Work out the finished part from the listing and answer in its coordinate system (mm). A direction names the side the tool comes from. Give positions to 0.01 mm unless a question says otherwise; leave off trailing zeros. Write each loop counter-clockwise with the first axis right and the second up, starting at its lowest first coordinate (ties: lowest second). Pieces come first, ordered by that corner, then holes.
1) Find section A-A (y = -11). Determine the outline of the cut face in (x, z).
2) Find section B-B (x = -92). Determine the outline of the cut face in (y, z), plus the area to 3 significant figures.
3) Straight lines are drawn through the part: probe 1 along Y at (x, z) = (-18, -18); probe 2 along X at (y, z) = (-7, -22); probe 3 along X at (y, z) = (-15.5, -32). For each, find the intervals that lie inside material, in ascending order.
4) Given pin 1 Ø12 at (x, y) = (-22, -35) entering from -Z; pin 2 Ø6 at (x, z) = (-67.5, -25.5) entering from -Y; pin 3 Ø7.5 at (y, z) = (-14, -30.5) entering from +X; pin 4 Ø10.5 at (x, z) = (-27.72, -17.76) entering from +Y, each flat-ended and moving along its own axis, determine where each tip first touches the part or whether it passes through.
5) A tool of negligible diameter and unlimited length cuts with its end or side. For faces 4 (the face through (-107, -46, -29)), 5 (the face through (-60, -3, -22)), 6 (the face through (-47, 0, -28)), from which of +Z, -Z, +X, -X, +Y, -Y can it reach the whole face along a straight path? Write none if from no direction.
6) Determine the mould class of faces 1 (the face through (-70.77, -1.48, -29.35)), 2 (the face through (-15.8, -17.5, -21.7)), 3 (the face through (-104.204, -24, -29)) for opening direction Z: pulls with the +Z half, pulls with the -Z half, needs draft (parallel to the pull), parting line crosses it, or undercut.
Autodesk Inventor part; units mm, degrees
ref_plane "YZ Plane" through (0, 0, 0) normal (1, 0, 0) x (0, 1, 0)
ref_plane "XZ Plane" through (0, 0, 0) normal (0, 1, 0) x (-1, 0, 0)
ref_plane "XY Plane" through (0, 0, 0) normal (0, 0, 1) x (1, 0, 0)
sketch "Sketch1" plane through (0, 0, 0) normal (0, 1, 0) x (-1, 0, 0)
  circle A0 centre (92.6541, -28.2127) radius 6.05
  circle A1 centre (65.1803, -27.0368) radius 6.05
  circle A2 centre (45.4573, -23.7633) radius 6.05
  circle A3 centre (92.6541, -28.2127) radius 7.55
  circle A4 centre (65.1803, -27.0368) radius 7.55
  circle A5 centre (45.4573, -23.7633) radius 7.55
  circle A6 centre (92.6541, -28.2127) radius 4
  circle A7 centre (45.4573, -23.7633) radius 4
  line L0 (92.6541, -28.2127) -> (100.2041, -28.2127)
  line L1 (70.678, -35.6025) -> (39.5208, -30.4313)
  line L2 (60.2143, -34.3811) -> (122.676, -37.0546)
  line L3 (51.451, -33.7618) -> (1.5927, -16.8916)
  line L4 (51.8932, -17.9704) -> (4.2209, -1.8399)
  circle A8 centre (27.7249, -17.7633) radius 4
  circle A9 centre (27.7249, -17.7633) radius 6.05
  circle A10 centre (27.7249, -17.7633) radius 7.55
  line L5 (27.7249, -17.7633) -> (20.1749, -17.7633)
  line L6 (20.1749, -17.7633) -> (16.1749, -17.7633)
  line L7 (16.1749, -17.7633) -> (10.1749, -17.7633)
  line L8 (10.1749, -17.7633) -> (10.1749, -19.7955)
  line L9 (10.1749, -19.7955) -> (10.1749, -3.8545)
  line L10 (13.1749, -17.7633) -> (13.1749, -20.8106)
  line L11 (13.1749, -20.8106) -> (13.1749, -4.8696)
  line L12 (13.1749, -20.8106) -> (13.1749, -16.8106)
  line L13 (13.1749, -4.8696) -> (13.1749, -8.8696)
  circle A11 centre (13.1749, -16.8106) radius 1
  circle A12 centre (13.1749, -8.8696) radius 1
  line L14 (16.1749, -17.7633) -> (16.1749, -21.8257)
  line L15 (16.1749, -17.7633) -> (16.1749, -5.8847)
  line L16 (114.6217, -21.596) -> (60.8612, -19.295)
  line L17 (100.2041, -28.2127) -> (104.2041, -28.2127)
  line L18 (104.2041, -28.2127) -> (110.2041, -28.2127)
  line L19 (107.2041, -28.2127) -> (107.2041, -21.2785)
  line L20 (107.2041, -28.2127) -> (107.2041, -36.3923)
  line L21 (107.2041, -36.3923) -> (107.2041, -28.3923)
  line L22 (107.2041, -21.2785) -> (107.2041, -25.2785)
  circle A13 centre (107.2041, -32.3923) radius 1
  circle A14 centre (107.2041, -25.2785) radius 1
  line L23 (110.2041, -28.2127) -> (110.2041, -36.5208)
  line L24 (104.2041, -28.2127) -> (104.2041, -36.2639)
  line L25 (104.2041, -28.2127) -> (104.2041, -21.1501)
  line L26 (110.2041, -28.2127) -> (110.2041, -21.4069)
  line L27 (75.2254, -21.0507) -> (39.3363, -15.0941)
  line L28 (65.1803, -27.0368) -> (45.4573, -27.0368)
  line L29 (55.3188, -33.0533) -> (55.3188, -17.7467)
  circle A15 centre (55.3188, -25.4) radius 1
  circle A16 centre (55.3188, -25.4) radius 2.55
  circle A17 centre (65.1803, -27.0368) radius 4
  point P0 (43.6173, -31.1112)
  point P1 (64.3979, -34.5602)
  point P2 (65.9627, -19.5133)
  point P3 (66.4165, -19.5886)
  point P4 (65.5031, -19.4937)
  point P5 (47.2973, -16.4154)
  point P6 (47.8772, -16.6116)
  point P7 (46.6935, -16.3152)
  dimension "d143" = 15.1
  dimension "d132" = 12.1
  dimension "d133" = 12.1
  dimension "d134" = 12.1
  dimension "d135" = 15.1
  dimension "d136" = 15.1
  dimension "d137" = 8
  dimension "d139" = 8
  dimension "d140" = 1.1759
  dimension "d141" = 3.2735
  dimension "d142" = 12.1
  dimension "d144" = 8
  dimension "d145" = 6
  dimension "d146" = 4
  dimension "d147" = 6
  dimension "d148" = 4
  dimension "d149" = 4
  dimension "d150" = 2
  dimension "d151" = 2
  dimension "d152" = 4
  dimension "d153" = 6
  dimension "d154" = 4
  dimension "d155" = 4
  dimension "d156" = 2
  dimension "d157" = 2
  dimension "d159" = 5.1
  dimension "d160" = 2
  dimension "d161" = 8
extrude "Extrusion1" add sketch "Sketch1" against normal blind 3 contours A3 | A3 L16 L25 L17 | L17 L24 L2 A3 | A3 L2 A4 L27 L16 | L27 A4 L16 | L16 A4 A16 L29 L27 | L2 L1 A4 | A4 A16 | L29 A16 A5 L4 L27 | L1 L29 A16 L28 A4 | A16 A4 | A4 A16 L28 L29 A15 | L27 A5 L3 A10 L4 | L4 A5 L27 | L29 A15 L28 A16 A5 | L28 A16 A4 | L1 A5 L28 A16 L29 | A5 A16 | A10 L6 L15 L4 | A10 | A15 L29 | L29 A15 | A5 A16 | A16 L29 L28 | L1 L3 A5 | A16 L28 L29 | A10 L3 L14 L6 | A16 L28 A5
extrude "Extrusion2" add sketch "Sketch1" along normal blind 0.5 contours A0 | A3 | A3 L16 L25 L17 | L17 L24 L2 A3 | A3 L2 A4 L27 L16 | L25 L16 L19 A14 L18 | L18 L20 A13 L2 L24 | L27 A4 L16 | L16 A4 A16 L29 L27 | L2 L1 A4 | A1 | A4 A16 | L19 A14 L16 L26 L18 | L18 L23 L2 L20 A13 | L29 A16 A5 L4 L27 | L1 L29 A16 L28 A4 | A16 A4 | A4 A16 L28 L29 A15 | L27 A5 L3 A10 L4 | L4 A5 L27 | L29 A15 L28 A16 A5 | L28 A16 A4 | L1 A5 L28 A16 L29 | A2 | A5 A16 | A10 L6 L15 L4 | A9 | A10 | A15 L29 | L29 A15 | A5 A16 | A16 L29 L28 | L1 L3 A5 | A16 L28 L29 | L15 L7 A11 L11 A12 L4 | A10 L3 L14 L6 | A16 L28 A5 | L11 A12 A11 L7 L9 L4 | L14 L3 L10 A11 L7 | L7 A11 L10 L3 L8
extrude "Extrusion8" add sketch "Sketch1" against normal blind 46 contours L25 L16 L19 A14 L18 | L18 L20 A13 L2 L24 | L19 A14 L16 L26 L18 | L18 L23 L2 L20 A13 | L15 L7 A11 L11 A12 L4 | L11 A12 A11 L7 L9 L4 | L14 L3 L10 A11 L7 | L7 A11 L10 L3 L8
extrude "Extrusion9" cut sketch "Sketch1" along normal through all both and the other way through all contours A15 L29 | L29 A15
properties part number "Servo Holder"
Results:
1. outline: (-110.2, -36.52) - (-104.2, -36.26) - (-104.2, -21.15) - (-110.2, -21.41) - close; (-16.17, -21.83) - (-10.17, -19.8) - (-10.17, -3.85) - (-16.17, -5.88) - close; hole circle Ø2 at (-107.2, -32.39); hole circle Ø2 at (-107.2, -25.28); hole circle Ø2 at (-13.17, -16.81); hole circle Ø2 at (-13.17, -8.87)
2. outline: (-3, -35.74) - (0.5, -35.74) - (0.5, -32.16) - (0, -32.16) - (0, -34.23) - (-3, -34.23) - close; (-3, -22.2) - (0, -22.2) - (0, -24.27) - (0.5, -24.27) - (0.5, -20.63) - (-3, -20.63) - close
2. area: 12.9 mm2
3. probe 1: y = -3 to 0.5
3. probe 2: x = -110.2 to -104.2
3. probe 3: x = -110.2 to -108.12, -106.28 to -104.2
4. pin 1: stops at z = -21.83
4. pin 2: stops at y = 0
4. pin 3: stops at x = -104.2
4. pin 4: stops at y = 0.5
5. face 4: +Z, -Z, +X, -X, -Y
5. face 5: +Z, -Z, -Y
5. face 6: -Y
6. face 1: undercut
6. face 2: pulls with the -Z half
6. face 3: needs draft
